Could you check a few things on this model? Use its own coordinates, in mm. Face numbers are marked on the shaded views. Give positions to 0.01 mm unless a question says otherwise; leave off trailing zeros. Loops run counter-clockwise (first coordinate to the right, second up) from the corner with the lowest first, then second, coordinate; pieces in that order, holes last. Notation, with made-up numbers: (16.5, 27.25) -> (45.5, 27.25) arc R16 cw to (45.5, 37.25) -> close; hole circle Ø10 at (-15, 32.5). An arc over 180 degrees is marked (long way). Write each question's results on one line, items separated by ' | '. Start each with the question number.
Q1. If we section it at B-B, the plane x = 48.5: List the corners of the cut face in (y, z) for me.
Q2. If we section it at C-C, the plane z = -6: Give the number of separate pieces and of enclosed holes in the cut face, plus the area to 3 significant figures.
Q3. We'd pull the mould along Y, two halves only. Please class the marked faces 1, 2, 3 and 4: released by +Y, released by -Y, zero draft, split by the parting line, or undercut.
Q4. If we section it at D-D, the plane x = 76: List the corners of the cut face in (y, z) for me, plus the area to 3 significant figures.
Q5. If I drill on line 1 along X through (y, z) = (17, -10); line 2 along X through (y, z) = (8.5, -2.5); line 3 along X through (y, z) = (26, -7.75), over which ranges is the centre line in solid material (lowest first)?
Q6. If we section it at A-A, the plane y = 28: List the corners of the cut face in (x, z) for me, plus the area to 3 significant figures.
Q7. Will this pin go through, and if not, where does the flat tip stop? P1, Ø12, axis at x = 64.5, y = 11, coming from the +Z side.
from build123d import *

# Parameters (mm, degrees)
F0_W     = 87.97396
F0_H     = 46.579894
F1_DEPTH = 10.8
F2_R     = 4.263815
F2_R_2   = 4.198962
F2_R_3   = 3.750182
F2_R_4   = 3.800158
F2_R_5   = 4.17849
F2_R_6   = 3.014974
F2_R_7   = 4.88964
F2_R_8   = 3.924494
F2_R_9   = 2.037287
F2_R_10  = 2.82101
F2_R_11  = 1.527268
F2_R_12  = 1.656553
F2_R_13  = 4.259792
F3_DEPTH = 25


with BuildPart() as f1:
    # F0 (on Top) → F1 (new body)
    with BuildSketch(Plane.XY):
        with Locations((43.98698, 23.289947)):
            Rectangle(F0_W, F0_H)
    extrude(amount=-F1_DEPTH)

    # F2 (on face) → F3 (cut)
    with BuildSketch(Plane.XY):
        with Locations((29.170312, 38.384426)):
            Circle(F2_R)
        with Locations((35.652604, 25.234634)):
            Circle(F2_R_2)
        with Locations((8.982603, 22.826925)):
            Circle(F2_R_3)
        with Locations((14.168437, 34.309842)):
            Circle(F2_R_4)
        with Locations((23.614062, 12.084842)):
            Circle(F2_R_5)
        with Locations((6.389686, 9.121509)):
            Circle(F2_R_6)
        with Locations((49.543228, 11.529217)):
            Circle(F2_R_3)
        with Locations((62.137399, 18.567134)):
            Circle(F2_R_7)
        with Locations((70.656978, 33.013385)):
            Circle(F2_R_8)
        with Locations((84.547602, 38.569633)):
            Circle(F2_R_9)
        with Locations((59.174061, 36.532342)):
            Circle(F2_R_10)
        with Locations((48.431981, 33.383802)):
            Circle(F2_R_11)
        with Locations((65.841563, 8.751092)):
            Circle(F2_R_12)
        with Locations((79.361774, 13.751717)):
            Circle(F2_R_13)
    extrude(amount=-F3_DEPTH, mode=Mode.SUBTRACT)


solid = f1.part
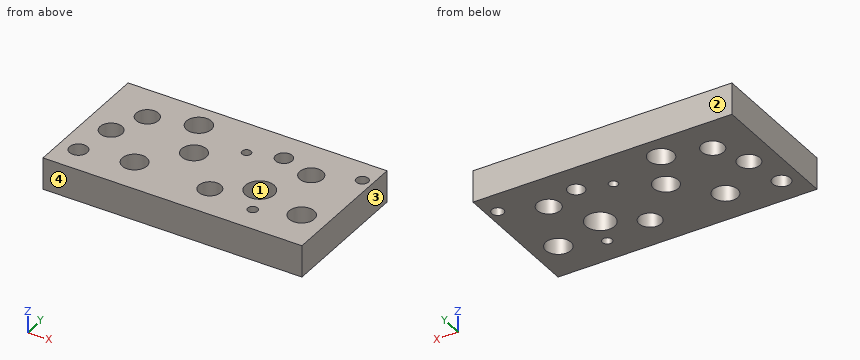
Final values:
1) outline: (0, -10.8) -> (7.93, -10.8) -> (7.93, 0) -> (0, 0) -> close; (15.13, -10.8) -> (31.86, -10.8) -> (31.86, 0) -> (15.13, 0) -> close; (34.91, -10.8) -> (46.58, -10.8) -> (46.58, 0) -> (34.91, 0) -> close
2) separate pieces: 1 | enclosed holes: 14 | area: 3,530 mm²
3) face 1: undercut | face 2: released by +Y | face 3: zero draft | face 4: released by -Y
4) outline: (0, -10.8) -> (11.14, -10.8) -> (11.14, 0) -> (0, 0) -> close; (16.37, -10.8) -> (46.58, -10.8) -> (46.58, 0) -> (16.37, 0) -> close | area: 447 mm²
5) line 1: x = 0 to 57.51, 66.77 to 76.61, 82.12 to 87.97 | line 2: x = 0 to 3.44, 9.34 to 21.47, 25.76 to 47.33, 51.75 to 64.2, 67.48 to 87.97 | line 3: x = 0 to 6.98, 10.98 to 31.52, 39.78 to 87.97
6) outline: (0, -10.8) -> (32.49, -10.8) -> (32.49, 0) -> (0, 0) -> close; (38.81, -10.8) -> (87.97, -10.8) -> (87.97, 0) -> (38.81, 0) -> close | area: 882 mm²
7) P1: stops at z = 0
